```python
from build123d import *

# Parameters (mm, degrees)
RESSALTO_EXTRUS_O1_DEPTH = 3
ESBO_O2_R                = 1.5
CORTE_EXTRUS_O1_DEPTH    = 23.869193252
FILETE1_R                = 5
FILETE2_R                = 2


with BuildPart() as part:
    # Esboço1 → Ressalto-extrusão1 (new body)
    with BuildSketch(Plane.XY):
        Polygon((0, 0), (4, 0), (4, 17), (11.2, 17), (11.2, 0), (15, 0), (15, -5), (0, -5), align=None)
    extrude(amount=RESSALTO_EXTRUS_O1_DEPTH)

    # Esboço2 → Corte-extrusão1 (cut, through all)
    with BuildSketch(Plane.XY.offset(3)):
        with Locations((7.6, 11.5)):
            Circle(ESBO_O2_R)
    extrude(amount=-CORTE_EXTRUS_O1_DEPTH, mode=Mode.SUBTRACT)

    # Filete1
    filete1_edges = [part.edges().sort_by_distance(p)[0] for p in [
        (0, -5, 1.5),
        (15, -5, 1.5),
    ]]
    fillet(filete1_edges, radius=FILETE1_R - 0.0001)  # a hair under: the kernel refuses the full size

    # Filete2
    filete2_edges = [part.edges().sort_by_distance(p)[0] for p in [
        (4, 17, 1.5),
        (11.2, 17, 1.5),
    ]]
    fillet(filete2_edges, radius=FILETE2_R)


solid = part.part
```
Part model, mm, in its own coordinate system. A direction names the side the tool comes from. Give positions to 0.01 mm unless a question says otherwise; leave off trailing zeros. Order: outer loops, then holes, each group sorted by start corner. A loop starts at its lowest first (then second) coordinate and runs counter-clockwise, first axis right, second up. Notation, with made-up numbers: (76, 26.5) - (96, 26.5) arc R23 ccw to (96, 46.5) - close; hole circle Ø3 at (-16.5, 19). An arc over 180 degrees is marked (long way). Use one line per item in the form item = value.
Item 1: Slice it at D-D on y = 5.25. Give the cut face in (x, z), and give its area (3 significant figures).
Solution:
outline = (4, 0) - (11.2, 0) - (11.2, 3) - (4, 3) - close
area = 21.6 mm2
Item 2: Two-plate mould, pull along Y, no slides. Class faces 4 (the face through (4.57, 16.4, 1.52)), 5 (the face through (8.986, 10.925, 1.521)), 6 (the face through (11.2, 8, 1)): released by +Y, released by -Y, zero draft, split by the parting line, or undercut.
Solution:
face_4 = released by +Y
face_5 = undercut
face_6 = zero draft
Item 3: Pin check, flat tips, straight feed: pin 1 Ø0.9 at (y, z) = (7.5, 1) entering from +X; pin 2 Ø2.5 at (x, y) = (7.6, 11.5) entering from +Z; pin 3 Ø0.9 at (x, z) = (2.5, 2) entering from +Y. Stop position of each tip, or through.
Solution:
pin_1 = 11.2
pin_2 = through
pin_3 = 0
Item 4: Probe probe 1 along Y at (x, z) = (7.6, 1.05); probe 2 along X at (y, z) = (14.5, 1.5); probe 3 along X at (y, z) = (10.5, 1.3). List the from-to ranges inside material, lowest first. Write a range as from..to.
Solution:
probe_1 = -5..10, 13..17
probe_2 = 4..11.2
probe_3 = 4..6.48, 8.72..11.2
Item 5: Slice it at B-B on x = 7.6. Give the cut face in (y, z).
Solution:
outline = (-5, 0) - (10, 0) - (10, 3) - (-5, 3) - close; (13, 0) - (17, 0) - (17, 3) - (13, 3) - close
Item 6: Which spindle directions (+Z, -Z, +X, -X, +Y, -Y) get a long thin tool onto all of the face, cutting with end or side? Do faces 1 (the face through (2, 0, 1)), 2 (the face through (13, 0, 1)), 3 (the face through (8, -5, 1)). Say none if no direction does.
Solution:
face_1 = +Z, -Z, -X, +Y
face_2 = +Z, -Z, +X, +Y
face_3 = +Z, -Z, +X, -X, -Y
Item 7: Slice it at A-A on y = 11.5. Give the cut face in (x, z), and give its area (3 significant figures).
Solution:
outline = (4, 0) - (6.1, 0) - (6.1, 3) - (4, 3) - close; (9.1, 0) - (11.2, 0) - (11.2, 3) - (9.1, 3) - close
area = 12.6 mm2
